Design review of the part built by this model. Coordinates are the model's own, in mm. A direction names the side the tool comes from. Coordinates: 2 decimals unless noted, no trailing zeros. Write each loop counter-clockwise with the first axis right and the second up, starting at its lowest first coordinate (ties: lowest second). Pieces come first, ordered by that corner, then holes. Notation, with made-up numbers: M 14.5,48 L 67.5,48 A26 ccw 67.5,69 Z; hole C 64.5,46.5 d11. An arc over 180 degrees is marked long. Write each question's results on one line, items separated by ' | '. Start each with the question number.
```python
from build123d import *

# Parameters (mm, degrees)
F1_DEPTH    = 3.4
F2_W        = 9
F2_H        = 9.8
F3_DEPTH    = 1
F4_W        = 9.0031104628
F4_H        = 9.8
F5_DEPTH    = 5
F7_D        = 3.1
F8_T1_DEPTH = 20.0867319519
F8_T3_DEPTH = 19.2898424147


# Not quite as in the source:
# - a fillet or chamfer that OpenCascade refuses, or shapes differently, is made with other operations: its cross-section is extruded or revolved along the edge and cut away or added


with BuildPart() as f1:
    # F0 (on Front) → F1 (new body)
    with BuildSketch(Plane.XZ):
        with BuildLine():
            Line((2.8, 0), (0, 0))
            Line((0, 0), (0, -9.8))
            ThreePointArc((0, -9.8), (1.4, -11.2), (2.8, -9.8))
            Line((2.8, -9.8), (2.8, 0))
        make_face()
    extrude(amount=F1_DEPTH)

    # F2 (on face) → F3 (join)
    with BuildSketch(Plane.XZ.offset(3.4)):
        with Locations((1.4, -4.9)):
            Rectangle(F2_W, F2_H)
    extrude(amount=F3_DEPTH)

    # F4 (on face) → F5 (join)
    with BuildSketch(Plane(origin=(0, 0, 0), x_dir=(-1, 0, 0), z_dir=(0, 1, 0))):
        with Locations((-1.4576160967, -4.9)):
            Rectangle(F4_W, F4_H)
    extrude(amount=F5_DEPTH)

    # F7 (through all)
    with Locations(Plane.XY):
        with Locations((1.4576160967, 2.5)):
            Hole(F7_D / 2)

    # F8: chamfer of 2 on 3 edges, made by hand

    # F8_s2 → F8_t1 (cut)
    with BuildSketch(Plane.XY.offset(-14.9433659759)):
        Polygon((-1.0439391347, 5), (-3.0439391347, 3), (-3.0439391347, 5), align=None)
        Polygon((5.9591713281, 3), (3.9591713281, 5), (5.9591713281, 5), align=None)
    extrude(amount=F8_T1_DEPTH, mode=Mode.SUBTRACT)

    # F8_s4 → F8_t3 (cut)
    with BuildSketch(Plane.YZ.offset(-8.1873051107)):
        Polygon((5, -7.8), (3, -9.8), (5, -9.8), align=None)
    extrude(amount=F8_T3_DEPTH, mode=Mode.SUBTRACT)


solid = f1.part
```
Item 1: Draft analysis for pull direction Y (two halves, no side actions). For faces 5 (the flat face through (1, 5, -4)), 6 (the cylindrical face through (1.4, -1.7, -11.2)), 7 (the flat face through (-2, 0, -5)), state which applies: released by +Y, released by -Y, zero draft, split by the parting line, or undercut.
Item 2: We need section C-C on z = -8.25. State the section outline as (x, y) points.
Item 3: Wall thickness on L1, parallel to X at y = 2.5, z = -5.75; L2, parallel to Y at x = 5, z = -1.5; L3, parallel to Y at x = 4.25, z = -8.75: over which ranges is each line inside the solid? List them lowest first.
Item 4: We need section A-A on x = -0.5. State the section outline as (y, z) points, then the cut area to 3 significant figures.
Item 5: We need section B-B on y = 2.5. State the section outline as (x, z) points, then the cut area to 3 significant figures.
Item 6: We need section D-D on x = 4.5. State the section outline as (y, z) points.
Item 7: Insertion check: pin 1 Ø0.9 at (x, y) = (3, 1) entering from -Z; pin 2 Ø1.1 at (y, z) = (-4, -5.5) entering from +X; pin 3 Ø1 at (y, z) = (-1, -6.5) entering from -X; pin 4 Ø1.5 at (x, z) = (1.5, -10.5) entering from -Y. Each pin has a flat end and moves straight along its axis. Give the tip position at first contact, or say it passes through.
Item 8: For faces 1 (the flat face through (1.5, 0.8, -9.8)), 2 (the flat face through (4, -3.4, -5)), 3 (the flat face through (0, -2, -5)), 4 (the flat face through (1, -3.4, -10)), list the 3-axis set-ups (+Z, -Z, +X, -X, +Y, -Y) from which the entire face can be reached by the end or side of a thin tool; tool diameter is ignored.
Answer:
1) face 5: released by +Y | face 6: zero draft | face 7: undercut
2) outline: M -3.1,-4.4 L 5.9,-4.4 L 5.9,-3.4 L 2.8,-3.4 L 2.8,0 L 5.96,0 L 5.96,3 L 4.41,4.55 L -1.49,4.55 L -3.04,3 L -3.04,0 L 0,0 L 0,-3.4 L -3.1,-3.4 Z; hole C 1.46,2.5 d3.1
3) L1: x = -3.04 to -0.09, 3.01 to 5.96 | L2: y = -4.4 to -3.4, 0 to 3.96 | L3: y = -4.4 to -3.4, 0 to 4.05
4) outline: M -4.4,-9.8 L -3.4,-9.8 L -3.4,0 L -4.4,0 Z; M 0,-9.8 L 3,-9.8 L 5,-7.8 L 5,0 L 0,0 Z | area: 56.8 mm^2
5) outline: M -3.04,-9.8 L -0.09,-9.8 L -0.09,0 L -3.04,0 Z; M 3.01,-9.8 L 5.96,-9.8 L 5.96,0 L 3.01,0 Z | area: 57.9 mm^2
6) outline: M -4.4,-9.8 L -3.4,-9.8 L -3.4,0 L -4.4,0 Z; M 0,-9.8 L 3,-9.8 L 4.46,-8.34 L 4.46,0 L 0,0 Z
7) pin 1: stops at z = -9.8 | pin 2: stops at x = 5.9 | pin 3: stops at x = 0 | pin 4: stops at y = -4.4
8) face 1: -Z, +X, -X, +Y | face 2: +Z, -Z, +X | face 3: +Z, -Z, -X | face 4: -Z, +X, -X, -Y
